Work out the finished part from the listing and answer in its coordinate system (mm). A direction names the side the tool comes from. Coordinates: 2 decimals unless noted, no trailing zeros. Loops run counter-clockwise (first coordinate to the right, second up) from the corner with the lowest first, then second, coordinate; pieces in that order, holes last.
```python
from build123d import *

# Parameters (mm, degrees)
SALIENTE_EXTRUIR1_DEPTH = 14
CROQUIS3_W              = 18
CROQUIS3_H              = 7.391109276
CORTAR_EXTRUIR1_DEPTH   = 83.825116963


with BuildPart() as part:
    # Croquis1 → Saliente-Extruir1 (new, symmetric)
    with BuildSketch(Plane.XY):
        Polygon((42, 0), (-42, 0), (-42, 14), (-31, 14), (-20, 70), (20, 70), (31, 14), (42, 14), align=None)
    extrude(amount=SALIENTE_EXTRUIR1_DEPTH, both=True)

    # Croquis3 → Cortar-Extruir1 (cut, through all)
    with BuildSketch(Plane(origin=(0, 70, 0), x_dir=(1, 0, 0), z_dir=(0, 1, 0))):
        with Locations((0, 10.304445362)):
            Rectangle(CROQUIS3_W, CROQUIS3_H)
        with Locations((0, -10.304445362)):
            Rectangle(CROQUIS3_W, CROQUIS3_H)
    extrude(amount=-CORTAR_EXTRUIR1_DEPTH, mode=Mode.SUBTRACT)


solid = part.part
```
1. Straight lines are drawn through the part: probe 1 along X at (y, z) = (54, -11.5); probe 2 along Z at (x, y) = (2, 10.5); probe 3 along Y at (x, z) = (38.5, 6.75). For each, find the intervals that lie inside material, in ascending order.
2. A cutting plane is placed at B-B, the plane y = 28. Give the vertices of the cut face in (x, z), then the cut area to 3 significant figures.
3. For faces 1 (the flat face through (-9, 35, -10)), 2 (the flat face through (-37, 14, 0)), 3 (the flat face through (36, 14, 0)), determine the directions among +Z, -Z, +X, -X, +Y, -Y from which every point of the face is accessible in a straight line to the end or side of a thin tool.
4. A cutting plane is placed at C-C, the plane z = -2.25. Give the vertices of the cut face in (x, y).
5. A cutting plane is placed at D-D, the plane x = -24. Give the vertices of the cut face in (y, z).
6. Determine the mould class of faces 4 (the flat face through (-22, 28, 14)), 5 (the flat face through (-25.577, 41.608, 0.196)), 6 (the flat face through (-9, 35, 10)) for opening direction X: released by +X, released by -X, zero draft, split by the parting line, or undercut.
7. Each of these flat-tipped pins is pushed along its axis until it touches: P1, Ø3, axis at x = -6, y = 39, coming from the +Z side; P2, Ø1.5, axis at y = 52, z = -1.5, coming from the -X side; P3, Ø2, axis at y = 26.5, z = -9, coming from the +X side; P4, Ø20, axis at x = 1, y = 40.5, coming from the -Z side. Where does it stop, or does it pass through?
8. A cutting plane is placed at A-A, the plane z = -11. Give the vertices of the cut face in (x, y), then the cut area to 3 significant figures.
Answers below:
1. probe 1: x = -23.14 to -9, 9 to 23.14
1. probe 2: z = -6.61 to 6.61
1. probe 3: y = 0 to 14
2. outline: (-28.25, -14) - (-9, -14) - (-9, -6.61) - (9, -6.61) - (9, -14) - (28.25, -14) - (28.25, 14) - (9, 14) - (9, 6.61) - (-9, 6.61) - (-9, 14) - (-28.25, 14) - close
2. area: 1,320 mm2
3. face 1: -Z, +Y, -Y
3. face 2: +Z, -Z, -X, +Y
3. face 3: +Z, -Z, +X, +Y
4. outline: (-42, 0) - (42, 0) - (42, 14) - (31, 14) - (20, 70) - (-20, 70) - (-31, 14) - (-42, 14) - close
5. outline: (0, -14) - (49.64, -14) - (49.64, 14) - (0, 14) - close
6. face 4: zero draft
6. face 5: released by -X
6. face 6: undercut
7. P1: stops at z = 6.61
7. P2: stops at x = -23.68
7. P3: stops at x = 28.74
7. P4: stops at z = -14
8. outline: (-42, 0) - (-9, 0) - (-9, 70) - (-20, 70) - (-31, 14) - (-42, 14) - close; (9, 0) - (42, 0) - (42, 14) - (31, 14) - (20, 70) - (9, 70) - close
8. area: 2,770 mm2
